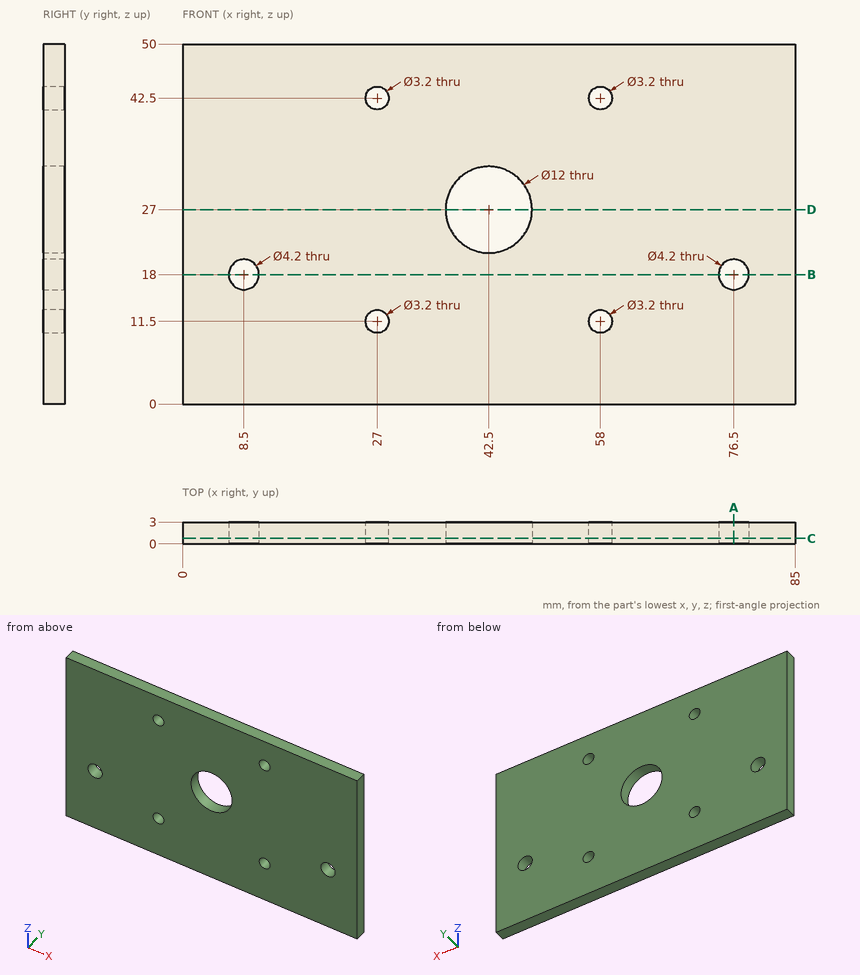
Input: dimensioned drawing with shaded views. Units: mm. Origin: part minimum x, y, z. Give positions to 0.01 mm unless a question says otherwise; leave off trailing zeros. Write each loop counter-clockwise with the first axis right and the second up, starting at its lowest first coordinate (ties: lowest second). Pieces come first, ordered by that corner, then holes. Notation, with made-up numbers: M 16.5,29 L 71.5,29 A36 cw 71.5,67 Z; hole C 48,-8 d4. An arc over 180 degrees is marked long. Return JSON: item names as keys, results as strings. Group by question number.
1) Material intervals for line 1 along X through (y, z) = (1.3, 42.5); line 2 along Z through (x, y) = (76.5, 1.35); line 3 along X through (y, z) = (2.25, 43.5), sorted ascending. Write a range as [from, to].
2) Cut plane D-D, the plane z = 27. Output: boundary loops of the cut face in (x, y), plus the area to 3 significant figures.
3) Pin query (flat end, axial travel): P1, Ø6, axis at x = 55, z = 16, coming from the -Y side. Return the tip coordinate at first contact, or that it passes through.
4) Cut plane A-A, the plane x = 76.5. Output: boundary loops of the cut face in (y, z).
5) Cut plane C-C, the plane y = 0.75. Output: boundary loops of the cut face in (x, z).
6) Cut plane B-B, the plane z = 18. Output: boundary loops of the cut face in (x, y), plus the area to 3 significant figures.
Recorded:
{
 "1": {"line 1": "x = [0, 25.4], [28.6, 56.4], [59.6, 85]", "line 2": "z = [0, 15.9], [20.1, 50]", "line 3": "x = [0, 25.75], [28.25, 56.75], [59.25, 85]"},
 "2": {"outline": "M 0,0 L 36.5,0 L 36.5,3 L 0,3 Z; M 48.5,0 L 85,0 L 85,3 L 48.5,3 Z", "area": "219 mm²"},
 "3": {"P1": "stops at y = 0"},
 "4": {"outline": "M 0,0 L 3,0 L 3,15.9 L 0,15.9 Z; M 0,20.1 L 3,20.1 L 3,50 L 0,50 Z"},
 "5": {"outline": "M 0,0 L 85,0 L 85,50 L 0,50 Z; hole C 8.5,18 d4.2; hole C 27,11.5 d3.2; hole C 27,42.5 d3.2; hole C 42.5,27 d12; hole C 58,11.5 d3.2; hole C 58,42.5 d3.2; hole C 76.5,18 d4.2"},
 "6": {"outline": "M 0,0 L 6.4,0 L 6.4,3 L 0,3 Z; M 10.6,0 L 74.4,0 L 74.4,3 L 10.6,3 Z; M 78.6,0 L 85,0 L 85,3 L 78.6,3 Z", "area": "230 mm²"}
}
